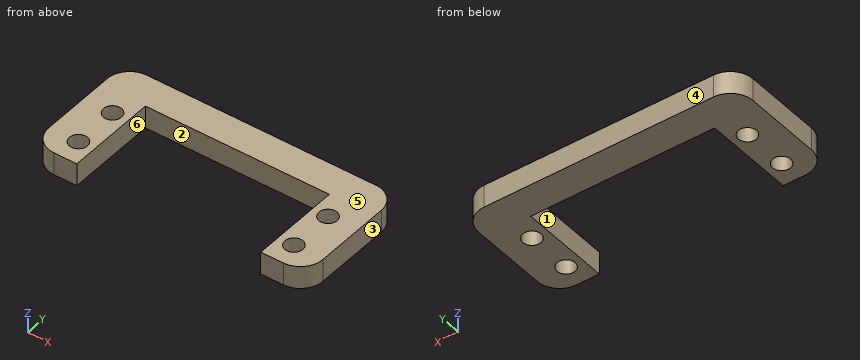
from build123d import *

# Parameters (mm, degrees)
SKETCH1_R           = 2
BOSS_EXTRUDE1_DEPTH = 5


with BuildPart() as part:
    # Sketch1 → Boss-Extrude1 (new body)
    with BuildSketch(Plane(origin=(0, 0, 0), x_dir=(0, 1, 0), z_dir=(0, 0, 1))):
        with BuildLine():
            Line((-10.05, 20.35), (10.05, 20.35))
            Line((10.05, 20.35), (10.05, -20.35))
            Line((10.05, -20.35), (-10.05, -20.35))
            Line((-10.05, -20.35), (-10.05, -25.35))
            ThreePointArc((-10.05, -25.35), (-8.585533906, -28.885533906), (-5.05, -30.35))
            Line((-5.05, -30.35), (12.05, -30.35))
            ThreePointArc((12.05, -30.35), (15.585533906, -28.885533906), (17.05, -25.35))
            Line((17.05, -25.35), (17.05, 25.35))
            ThreePointArc((17.05, 25.35), (15.585533906, 28.885533906), (12.05, 30.35))
            Line((12.05, 30.35), (-5.05, 30.35))
            ThreePointArc((-5.05, 30.35), (-8.585533906, 28.885533906), (-10.05, 25.35))
            Line((-10.05, 25.35), (-10.05, 20.35))
        make_face()
        with Locations(Location((5.05, 23.85, 0), (0, 0, 270))):
            Circle(SKETCH1_R, mode=Mode.SUBTRACT)
        with Locations(Location((-4.95, 23.85, 0), (0, 0, 270))):
            Circle(SKETCH1_R, mode=Mode.SUBTRACT)
        with Locations(Location((5.05, -23.85, 0), (0, 0, 90))):
            Circle(SKETCH1_R, mode=Mode.SUBTRACT)
        with Locations(Location((-4.95, -23.85, 0), (0, 0, 90))):
            Circle(SKETCH1_R, mode=Mode.SUBTRACT)
    extrude(amount=-BOSS_EXTRUDE1_DEPTH)


solid = part.part
Geometry: final body of the model. Coordinates: model frame, mm. Face numbers are marked on the shaded views. A direction names the side the tool comes from. Round coordinates to 2 decimals unless told otherwise and drop trailing zeros. Order: outer loops, then holes, each group sorted by start corner. A loop starts at its lowest first (then second) coordinate and runs counter-clockwise, first axis right, second up.
Q1. Section A-A, the plane y = 5.05. Output: boundary loops of the cut face in (x, z), and give its area (3 significant figures).
Result sheet:
outline: (-30.35, -5) - (-25.85, -5) - (-25.85, 0) - (-30.35, 0) - close; (-21.85, -5) - (-20.35, -5) - (-20.35, 0) - (-21.85, 0) - close; (20.35, -5) - (21.85, -5) - (21.85, 0) - (20.35, 0) - close; (25.85, -5) - (30.35, -5) - (30.35, 0) - (25.85, 0) - close
area: 60.0 mm2
Q2. Section B-B, the plane x = 23.85. Output: boundary loops of the cut face in (y, z), and give its area (3 significant figures).
Result sheet:
outline: (-10.05, -5) - (-6.95, -5) - (-6.95, 0) - (-10.05, 0) - close; (-2.95, -5) - (3.05, -5) - (3.05, 0) - (-2.95, 0) - close; (7.05, -5) - (17.05, -5) - (17.05, 0) - (7.05, 0) - close
area: 95.5 mm2
Q3. Section C-C, the plane z = -2.15. Output: boundary loops of the cut face in (x, y), and give its area (3 significant figures).
Result sheet:
outline: (-30.35, -5.05) arc R5 ccw to (-25.35, -10.05) - (-20.35, -10.05) - (-20.35, 10.05) - (20.35, 10.05) - (20.35, -10.05) - (25.35, -10.05) arc R5 ccw to (30.35, -5.05) - (30.35, 12.05) arc R5 ccw to (25.35, 17.05) - (-25.35, 17.05) arc R5 ccw to (-30.35, 12.05) - close; hole circle Ø4 at (-23.85, -4.95); hole circle Ø4 at (-23.85, 5.05); hole circle Ø4 at (23.85, -4.95); hole circle Ø4 at (23.85, 5.05)
area: 755 mm2
Q4. Mould query, pull axis X, two halves, no side actions, for the marked faces 1, 2, 3 and 4. Classes: released by +X, released by -X, zero draft, split by the parting line, or undercut.
Result sheet:
face 1: undercut
face 2: undercut
face 3: released by +X
face 4: zero draft
Q5. Access query for the marked faces 5 and 6. Directions: +Z, -Z, +X, -X, +Y, -Y. A direction counts if a zero-diameter tool reaches every point of the face in a straight line with its end or side. Return the directions, or none.
Result sheet:
face 5: +Z, +X, -X, +Y, -Y
face 6: +Z, -Z, -Y
Q6. Material intervals for probe 1 along Y at (x, z) = (-23.85, -0.95); probe 2 along X at (y, z) = (2, -1.7); probe 3 along Y at (x, z) = (24.5, -4.2), sorted ascending.
Result sheet:
probe 1: y = -10.05 to -6.95, -2.95 to 3.05, 7.05 to 17.05
probe 2: x = -30.35 to -20.35, 20.35 to 30.35
probe 3: y = -10.05 to -6.84, -3.06 to 3.16, 6.94 to 17.05
Q7. Pin query (flat end, axial travel): pin 1 (3.5 mm diameter, centred on x = 23.85, y = 5.05, fed in from -Z); pin 2 (1.5 mm diameter, centred on x = 1, z = -3.5, fed in from -Y). Return the tip coordinate at first contact, or that it passes through.
Result sheet:
pin 1: passes through
pin 2: stops at y = 10.05
Q8. Section D-D, the plane x = -17.5. Output: boundary loops of the cut face in (y, z).
Result sheet:
outline: (10.05, -5) - (17.05, -5) - (17.05, 0) - (10.05, 0) - close
